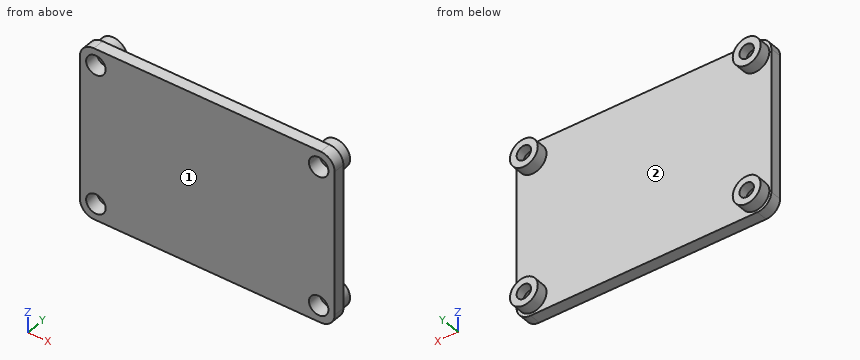
from build123d import *

# Parameters (mm, degrees)
SKETCH_1_R          = 1.55
EXTRUDE_1_DEPTH     = 2.5
SKETCH_2_R          = 3
EXTRUDE_2_DEPTH     = 2.5
SKETCH_3_R          = 1.55
CUT_EXTRUDE_1_DEPTH = 34.466573357
SKETCH_4_R          = 2.1
CUT_EXTRUDE_2_DEPTH = 3


with BuildPart() as part:
    # Sketch 1 → Extrude 1 (new body)
    with BuildSketch(Plane(origin=(0, 0, 0), x_dir=(1, 0, 0), z_dir=(0, 1, 0))):
        with BuildLine():
            Line((-27.4365, 0), (-27.4365, 15.5))
            ThreePointArc((-27.4365, 15.5), (-26.557820344, 17.621320344), (-24.4365, 18.5))
            Line((-24.4365, 18.5), (0, 18.5))
            Line((0, 18.5), (24.4365, 18.5))
            ThreePointArc((24.4365, 18.5), (26.557820344, 17.621320344), (27.4365, 15.5))
            Line((27.4365, 15.5), (27.4365, 0))
            Line((27.4365, 0), (27.4365, -15.5))
            ThreePointArc((27.4365, -15.5), (26.557820344, -17.621320344), (24.4365, -18.5))
            Line((24.4365, -18.5), (0, -18.5))
            Line((0, -18.5), (-24.4365, -18.5))
            ThreePointArc((-24.4365, -18.5), (-26.557820344, -17.621320344), (-27.4365, -15.5))
            Line((-27.4365, -15.5), (-27.4365, 0))
        make_face()
        with Locations(Location((-24, 15, 0), (0, 0, 270))):
            Circle(SKETCH_1_R, mode=Mode.SUBTRACT)
        with Locations(Location((24, 15, 0), (0, 0, 270))):
            Circle(SKETCH_1_R, mode=Mode.SUBTRACT)
        with Locations(Location((24, -15, 0), (0, 0, 90))):
            Circle(SKETCH_1_R, mode=Mode.SUBTRACT)
        with Locations(Location((-24, -15, 0), (0, 0, 90))):
            Circle(SKETCH_1_R, mode=Mode.SUBTRACT)
    extrude(amount=EXTRUDE_1_DEPTH)

    # Sketch 2 → Extrude 2 (add)
    with BuildSketch(Plane(origin=(0, 2.5, 0), x_dir=(1, 0, 0), z_dir=(0, 1, 0))):
        with Locations(Location((-24, 15, 0), (0, 0, 270))):
            Circle(SKETCH_2_R)
        with Locations(Location((24, 15, 0), (0, 0, 270))):
            Circle(SKETCH_2_R)
        with Locations(Location((-24, -15, 0), (0, 0, 270))):
            Circle(SKETCH_2_R)
        with Locations(Location((24, -15, 0), (0, 0, 270))):
            Circle(SKETCH_2_R)
    extrude(amount=EXTRUDE_2_DEPTH)

    # Sketch 3 → Cut-Extrude 1 (cut, through all)
    with BuildSketch(Plane.XZ):
        with Locations(Location((-24, 15, 0), (0, 0, 270))):
            Circle(SKETCH_3_R)
        with Locations(Location((24, 15, 0), (0, 0, 270))):
            Circle(SKETCH_3_R)
        with Locations(Location((-24, -15, 0), (0, 0, 270))):
            Circle(SKETCH_3_R)
        with Locations(Location((24, -15, 0), (0, 0, 270))):
            Circle(SKETCH_3_R)
    extrude(amount=-CUT_EXTRUDE_1_DEPTH, mode=Mode.SUBTRACT)

    # Sketch 4 → Cut-Extrude 2 (cut)
    with BuildSketch(Plane(origin=(0, 0, 0), x_dir=(-1, 0, 0), z_dir=(0, -1, 0))):
        with Locations(Location((24, -15, 0), (0, 0, 90))):
            Circle(SKETCH_4_R)
        with Locations(Location((-24, -15, 0), (0, 0, 90))):
            Circle(SKETCH_4_R)
        with Locations(Location((-24, 15, 0), (0, 0, 270))):
            Circle(SKETCH_4_R)
        with Locations(Location((24, 15, 0), (0, 0, 270))):
            Circle(SKETCH_4_R)
    extrude(amount=-CUT_EXTRUDE_2_DEPTH, mode=Mode.SUBTRACT)


solid = part.part
The listing builds one solid part. Answer for the finished solid, in the listing's coordinates (mm). Face numbers are marked on the shaded views. Coordinates: 2 decimals unless noted, no trailing zeros. Loops run counter-clockwise (first coordinate to the right, second up) from the corner with the lowest first, then second, coordinate; pieces in that order, holes last. Notation, with made-up numbers: (48.5, -5) -> (101.5, -5) arc R30 cw to (101.5, 18) -> close; hole circle Ø9 at (56.5, 20.25). An arc over 180 degrees is marked (long way). Answer in a Markdown table with one row per item. Add a question column.
1. The part is cut by section C-C, the plane x = -20. Write down the section's boundary in (y, z).
2. The part is cut by section A-A, the plane y = 4.4. Write down the section's boundary in (x, z), then the cut area to 3 significant figures.
3. Consider line 1 (X direction, y = 3.9, z = -15); line 2 (X direction, y = 1.6, z = 15); line 3 (X direction, y = 0.35, z = 14.5). Determine where each line is inside the solid, lowest interval first. Write a range as [from, to].
4. Determine the mould class of the marked faces 1 and 2 for opening direction Z: +Z half, -Z half, draft (parallel to the pull), parting line (faces both ways), or undercut.
5. The part is cut by section B-B, the plane y = 1.5. Write down the section's boundary in (x, z).
6. Flat-ended cylindrical pins translate along their axes: P1, Ø3, axis at x = 24, z = 15, coming from the -Y side; P2, Ø5, axis at x = -24, z = -15, coming from the -Y side; P3, Ø2, axis at x = 23, z = -15, coming from the -Y side; P4, Ø1, axis at x = -7, z = -9.5, coming from the +Y side. Find the tip coordinate at first contact, or state that the pin passes through.
Answer below:
| question | item | result |
|---|---|---|
| 1 | outline | (0, -18.5) -> (2.5, -18.5) -> (2.5, 18.5) -> (0, 18.5) -> close |
| 2 | outline | circle Ø6 at (-24, -15); circle Ø6 at (-24, 15); circle Ø6 at (24, -15); circle Ø6 at (24, 15); hole circle Ø3.1 at (-24, -15); hole circle Ø3.1 at (-24, 15); hole circle Ø3.1 at (24, -15); hole circle Ø3.1 at (24, 15) |
| 2 | area | 82.9 mm2 |
| 3 | line 1 | [-27, -25.55], [-22.45, -21], [21, 22.45], [25.55, 27] |
| 3 | line 2 | [-27.44, -26.1], [-21.9, 21.9], [26.1, 27.44] |
| 3 | line 3 | [-27.44, -26.04], [-21.96, 21.96], [26.04, 27.44] |
| 4 | face 1 | draft |
| 4 | face 2 | undercut |
| 5 | outline | (-27.44, -15.5) arc R3 ccw to (-24.44, -18.5) -> (24.44, -18.5) arc R3 ccw to (27.44, -15.5) -> (27.44, 15.5) arc R3 ccw to (24.44, 18.5) -> (-24.44, 18.5) arc R3 ccw to (-27.44, 15.5) -> close; hole circle Ø4.2 at (-24, -15); hole circle Ø4.2 at (-24, 15); hole circle Ø4.2 at (24, -15); hole circle Ø4.2 at (24, 15) |
| 6 | P1 | through |
| 6 | P2 | y = 0 |
| 6 | P3 | y = 3 |
| 6 | P4 | y = 2.5 |
